Can you work these out from the model? Positions are in its coordinate system, mm. A direction names the side the tool comes from. Round coordinates to 2 decimals unless told otherwise and drop trailing zeros. Loops run counter-clockwise (first coordinate to the right, second up) from the corner with the lowest first, then second, coordinate; pieces in that order, holes last. Notation, with made-up numbers: (34.5, 61) -> (77.5, 61) arc R26 cw to (77.5, 78) -> close; hole circle Ø9 at (-8, 51.25). An arc over 180 degrees is marked (long way). Write item = value, one per line.
from build123d import *

# Parameters (mm, degrees)
F0_R     = 46.3869587869
F7_DEPTH = 276.5972781926
F8_R     = 46.3869587869
F1_DEPTH = 25.4
F2_R     = 52.1237255929
F3_DEPTH = 325.6295006722
F4_W     = 132.3714181781
F4_H     = 167.2963500023
F5_DEPTH = 127
F9_DEPTH = 50.8


with BuildPart() as f7:
    # F0 (on Front) → F7 (new body)
    with BuildSketch(Plane.XZ):
        Circle(F0_R)
    extrude(amount=F7_DEPTH)

    # F8 (on face) → F1 (join)
    with BuildSketch(Plane.XZ.offset(276.5972781926)):
        with BuildLine():
            Line((482.9649029074, 16.5669820287), (16.2037538756, 69.9342963946))
            ThreePointArc((16.2037538756, 69.9342963946), (56.1986906588, 44.6662581834), (71.7869587869, 0))
            ThreePointArc((71.7869587869, 0), (56.2879281413, -44.5537495328), (16.4834153308, -69.8689091865))
            Line((16.4834153308, -69.8689091865), (482.9649029074, -15.5880084808))
            Line((482.9649029074, -15.5880084808), (482.9649029074, 16.5669820287))
        make_face()
        with BuildLine():
            Line((16.2037538756, 69.9342963946), (0, 71.7869587869))
            ThreePointArc((0, 71.7869587869), (-71.7869587869, 0), (0, -71.7869587869))
            Line((0, -71.7869587869), (16.4834153308, -69.8689091865))
            ThreePointArc((16.4834153308, -69.8689091865), (56.2879281413, -44.5537495328), (71.7869587869, 0))
            ThreePointArc((71.7869587869, 0), (56.1986906588, 44.6662581834), (16.2037538756, 69.9342963946))
        make_face()
        Circle(F8_R, mode=Mode.SUBTRACT)
        Circle(F8_R)
    extrude(amount=F1_DEPTH)

    # F2 (on face) → F3 (join)
    with BuildSketch(Plane.XZ.offset(301.9972781926)):
        Circle(F2_R)
    extrude(amount=F3_DEPTH)

    # F4 (on face) → F5 (join)
    with BuildSketch(Plane.XZ.offset(627.6267788649)):
        with Locations((-0.5969889462, 0.5796924233)):
            Rectangle(F4_W, F4_H)
    extrude(amount=F5_DEPTH)

    # F6 (on face) → F9 (join)
    with BuildSketch(Plane.XZ.offset(754.6267788649)):
        with BuildLine():
            Line((-0.5969889462, 107.3650692829), (55.9769339649, 85.7203485594))
            ThreePointArc((55.9769339649, 85.7203485594), (29.7297504424, 101.8741817091), (-0.5969889462, 107.3650692829))
        make_face()
        with BuildLine():
            ThreePointArc((70.9482696087, 67.6243206263), (64.1043554081, 77.2032748025), (55.9769339649, 85.7203485594))
            Line((55.9769339649, 85.7203485594), (-0.5969889462, 107.3650692829))
            Line((-0.5969889462, 107.3650692829), (70.9482696087, 67.6243206263))
        make_face()
        with BuildLine():
            Line((70.9482696087, 67.6243206263), (-0.5969889462, 107.3650692829))
            ThreePointArc((-0.5969889462, 107.3650692829), (-83.1992115072, 24.1679996252), (-0.5969889462, -59.0290700325))
            ThreePointArc((-0.5969889462, -59.0290700325), (58.6192791913, -34.8734172151), (83.1992115072, 24.1679996252))
            ThreePointArc((83.1992115072, 24.1679996252), (80.0779273104, 46.7430821962), (70.9482696087, 67.6243206263))
        make_face()
        with BuildLine():
            Line((823.5844914503, -350.4373025497), (70.9482696087, 67.6243206263))
            ThreePointArc((70.9482696087, 67.6243206263), (80.0779273104, 46.7430821962), (83.1992115072, 24.1679996252))
            ThreePointArc((83.1992115072, 24.1679996252), (58.6192791913, -34.8734172151), (-0.5969889462, -59.0290700325))
            Line((-0.5969889462, -59.0290700325), (823.5844914503, -350.4373025497))
        make_face()
    extrude(amount=F9_DEPTH)


solid = f7.part
1. We'd pull the mould along Y, two halves only. Please class faces 1 (the flat face through (405.72, -779.67, -202.69)), 2 (the cylindrical face through (-6.79, -462.53, 51.68)), 3 (the flat face through (-1, -754.627, 93)), 4 (the flat face through (-66.783, -690, -1)): released by +Y, released by -Y, zero draft, split by the parting line, or undercut.
Entries:
face_1 = zero draft
face_2 = undercut
face_3 = released by +Y
face_4 = undercut
2. For faces 5 (the cylindrical face through (-10.056, -136.362, -45.284)), 6 (the flat face through (302, -754.627, -121)), 7 (the cylindrical face through (-71.77, -289.12, 1.58)), which set-ups out of +Z, -Z, +X, -X, +Y, -Y let a thin tool reach every point of the face, with its end or its side?
Entries:
face_5 = +Y
face_6 = +Z, -Z, +X
face_7 = -X, +Y
3. I need wall thicknesses on line 1 (Y direction, x = 437, z = -160.5); line 2 (Y direction, x = 36.5, z = 68); line 3 (X direction, y = -725, z = 60). Which ranges of each line are inside material? Lowest first, please. Write a range as [from, to].
Entries:
line_1 = [-805.43, -754.63]
line_2 = [-805.43, -627.63]
line_3 = [-66.78, 65.59]
4. Suppose I cut it at C-C, the plane y = -738. List the corners of the cut face in (x, z) for me.
Entries:
outline = (-66.78, -83.07) -> (65.59, -83.07) -> (65.59, 84.23) -> (-66.78, 84.23) -> close
5. Suppose I cut it at B-B, the plane x = -26. List the corners of the cut face in (y, z) for me.
Entries:
outline = (-805.43, -54.86) -> (-754.63, -54.86) -> (-754.63, -83.07) -> (-627.63, -83.07) -> (-627.63, -45.18) -> (-302, -45.18) -> (-302, -66.91) -> (-276.6, -66.91) -> (-276.6, -38.42) -> (0, -38.42) -> (0, 38.42) -> (-276.6, 38.42) -> (-276.6, 66.91) -> (-302, 66.91) -> (-302, 45.18) -> (-627.63, 45.18) -> (-627.63, 84.23) -> (-754.63, 84.23) -> (-754.63, 103.2) -> (-805.43, 103.2) -> close
6. Suppose I cut it at A-A, the plane x = 372. List the corners of the cut face in (y, z) for me, and give its area (3 significant figures).
Entries:
outline = (-805.43, -190.77) -> (-754.63, -190.77) -> (-754.63, -99.6) -> (-805.43, -99.6) -> close; (-302, -28.5) -> (-276.6, -28.5) -> (-276.6, 29.25) -> (-302, 29.25) -> close
area = 6,100 mm²
7. I'm going to push flat-ended pins straight in: pin 1 (10 mm diameter, centred on x = 237, z = -93, fed in from +Y); pin 2 (3 mm diameter, centred on x = 8, y = -674, fed in from +Z); pin 3 (13 mm diameter, centred on x = -72, z = 40.5, fed in from +Y). Where does each tip first touch, or does it pass through?
Entries:
pin_1 = -754.63
pin_2 = 84.23
pin_3 = -627.63
8. Suppose I cut it at D-D, the plane z = 0. List the corners of the cut face in (x, y) for me.
Entries:
outline = (-79.61, -805.43) -> (192.69, -805.43) -> (192.69, -754.63) -> (65.59, -754.63) -> (65.59, -627.63) -> (52.12, -627.63) -> (52.12, -302) -> (482.96, -302) -> (482.96, -276.6) -> (46.39, -276.6) -> (46.39, 0) -> (-46.39, 0) -> (-46.39, -276.6) -> (-71.79, -276.6) -> (-71.79, -302) -> (-52.12, -302) -> (-52.12, -627.63) -> (-66.78, -627.63) -> (-66.78, -754.63) -> (-79.61, -754.63) -> close
